```python
from build123d import *

# Parameters (mm, degrees)
MODEL_R                 = 1.5
SALIENTE_EXTRUIR1_DEPTH = 3


with BuildPart() as part:
    # Model → Saliente-Extruir1 (new body)
    with BuildSketch(Plane.XY):
        with BuildLine():
            Line((-1383.727545355, 378.908179756), (-1386.727545355, 378.908179756))
            Line((-1386.727545355, 378.908179756), (-1386.727545355, 380.408179756))
            ThreePointArc((-1386.727545355, 380.408179756), (-1387.166885184, 381.468839928), (-1388.227545355, 381.908179756))
            Line((-1388.227545355, 381.908179756), (-1395.72785056, 381.908179756))
            ThreePointArc((-1395.72785056, 381.908179756), (-1396.788510732, 381.468839928), (-1397.22785056, 380.408179756))
            Line((-1397.22785056, 380.408179756), (-1469.22785056, 380.408179756))
            ThreePointArc((-1469.22785056, 380.408179756), (-1469.667190388, 381.468839928), (-1470.72785056, 381.908179756))
            Line((-1470.72785056, 381.908179756), (-1478.227545355, 381.908179756))
            ThreePointArc((-1478.227545355, 381.908179756), (-1479.288205527, 381.468839928), (-1479.727545355, 380.408179756))
            Line((-1479.727545355, 380.408179756), (-1479.727545355, 378.908179756))
            Line((-1479.727545355, 378.908179756), (-1482.727545355, 378.908179756))
            Line((-1482.727545355, 378.908179756), (-1482.727545355, 368.408179756))
            Line((-1482.727545355, 368.408179756), (-1473.852545355, 368.408179756))
            Line((-1473.852545355, 368.408179756), (-1473.852545355, 369.658179757))
            ThreePointArc((-1473.852545355, 369.658179757), (-1473.632875441, 370.188509842), (-1473.102545355, 370.408179756))
            Line((-1473.102545355, 370.408179756), (-1471.352545355, 370.408179756))
            ThreePointArc((-1471.352545355, 370.408179756), (-1470.82221527, 370.188509842), (-1470.602545355, 369.658179757))
            Line((-1470.602545355, 369.658179757), (-1470.602545355, 368.408179756))
            Line((-1470.602545355, 368.408179756), (-1466.977545355, 368.408179756))
            ThreePointArc((-1466.977545355, 368.408179756), (-1466.44721527, 368.188509842), (-1466.227545355, 367.658179756))
            Line((-1466.227545355, 367.658179756), (-1466.227545355, 366.158179756))
            ThreePointArc((-1466.227545355, 366.158179756), (-1466.44721527, 365.627849671), (-1466.977545355, 365.408179756))
            Line((-1466.977545355, 365.408179756), (-1470.602545355, 365.408179756))
            Line((-1470.602545355, 365.408179756), (-1470.602545355, 364.158179756))
            ThreePointArc((-1470.602545355, 364.158179756), (-1470.82221527, 363.627849671), (-1471.352545355, 363.408179756))
            Line((-1471.352545355, 363.408179756), (-1473.102545355, 363.408179756))
            ThreePointArc((-1473.102545355, 363.408179756), (-1473.632875441, 363.627849671), (-1473.852545355, 364.158179756))
            Line((-1473.852545355, 364.158179756), (-1473.852545355, 365.408179756))
            Line((-1473.852545355, 365.408179756), (-1482.727545355, 365.408179756))
            Line((-1482.727545355, 365.408179756), (-1482.727545355, 350.408179756))
            Line((-1482.727545355, 350.408179756), (-1473.852545355, 350.408179756))
            Line((-1473.852545355, 350.408179756), (-1473.852545355, 351.658179756))
            ThreePointArc((-1473.852545355, 351.658179756), (-1473.632875441, 352.188509842), (-1473.102545355, 352.408179756))
            Line((-1473.102545355, 352.408179756), (-1471.352545355, 352.408179756))
            ThreePointArc((-1471.352545355, 352.408179756), (-1470.82221527, 352.188509842), (-1470.602545355, 351.658179756))
            Line((-1470.602545355, 351.658179756), (-1470.602545355, 350.408179756))
            Line((-1470.602545355, 350.408179756), (-1466.977545355, 350.408179756))
            ThreePointArc((-1466.977545355, 350.408179756), (-1466.44721527, 350.188509842), (-1466.227545355, 349.658179756))
            Line((-1466.227545355, 349.658179756), (-1466.227545355, 348.158179756))
            ThreePointArc((-1466.227545355, 348.158179756), (-1466.44721527, 347.627849671), (-1466.977545355, 347.408179756))
            Line((-1466.977545355, 347.408179756), (-1470.602545355, 347.408179756))
            Line((-1470.602545355, 347.408179756), (-1470.602545355, 346.158179756))
            ThreePointArc((-1470.602545355, 346.158179756), (-1470.82221527, 345.627849671), (-1471.352545355, 345.408179756))
            Line((-1471.352545355, 345.408179756), (-1473.102545355, 345.408179756))
            ThreePointArc((-1473.102545355, 345.408179756), (-1473.632875441, 345.627849671), (-1473.852545355, 346.158179756))
            Line((-1473.852545355, 346.158179756), (-1473.852545355, 347.408179756))
            Line((-1473.852545355, 347.408179756), (-1482.727545355, 347.408179756))
            Line((-1482.727545355, 347.408179756), (-1482.727545355, 336.908179756))
            Line((-1482.727545355, 336.908179756), (-1479.727545355, 336.908179756))
            Line((-1479.727545355, 336.908179756), (-1479.727545355, 335.408179756))
            ThreePointArc((-1479.727545355, 335.408179756), (-1479.288205527, 334.347519585), (-1478.227545355, 333.908179756))
            Line((-1478.227545355, 333.908179756), (-1470.72785056, 333.908179756))
            ThreePointArc((-1470.72785056, 333.908179756), (-1469.667190388, 334.347519585), (-1469.22785056, 335.408179756))
            Line((-1469.22785056, 335.408179756), (-1397.22785056, 335.408179756))
            ThreePointArc((-1397.22785056, 335.408179756), (-1396.788510732, 334.347519585), (-1395.72785056, 333.908179756))
            Line((-1395.72785056, 333.908179756), (-1388.227545355, 333.908179756))
            ThreePointArc((-1388.227545355, 333.908179756), (-1387.166885184, 334.347519585), (-1386.727545355, 335.408179756))
            Line((-1386.727545355, 335.408179756), (-1386.727545355, 336.908179756))
            Line((-1386.727545355, 336.908179756), (-1383.727545355, 336.908179756))
            Line((-1383.727545355, 336.908179756), (-1383.727545355, 347.408179756))
            Line((-1383.727545355, 347.408179756), (-1392.602545355, 347.408179756))
            Line((-1392.602545355, 347.408179756), (-1392.602545355, 346.158179756))
            ThreePointArc((-1392.602545355, 346.158179756), (-1392.82221527, 345.627849671), (-1393.352545355, 345.408179756))
            Line((-1393.352545355, 345.408179756), (-1395.102545355, 345.408179756))
            ThreePointArc((-1395.102545355, 345.408179756), (-1395.632875441, 345.627849671), (-1395.852545355, 346.158179756))
            Line((-1395.852545355, 346.158179756), (-1395.852545355, 347.408179756))
            Line((-1395.852545355, 347.408179756), (-1399.477545355, 347.408179756))
            ThreePointArc((-1399.477545355, 347.408179756), (-1400.007875441, 347.627849671), (-1400.227545355, 348.158179756))
            Line((-1400.227545355, 348.158179756), (-1400.227545355, 349.658179756))
            ThreePointArc((-1400.227545355, 349.658179756), (-1400.007875441, 350.188509842), (-1399.477545355, 350.408179756))
            Line((-1399.477545355, 350.408179756), (-1395.852545355, 350.408179756))
            Line((-1395.852545355, 350.408179756), (-1395.852545355, 351.658179756))
            ThreePointArc((-1395.852545355, 351.658179756), (-1395.632875441, 352.188509842), (-1395.102545355, 352.408179756))
            Line((-1395.102545355, 352.408179756), (-1393.352545355, 352.408179756))
            ThreePointArc((-1393.352545355, 352.408179756), (-1392.82221527, 352.188509842), (-1392.602545355, 351.658179756))
            Line((-1392.602545355, 351.658179756), (-1392.602545355, 350.408179756))
            Line((-1392.602545355, 350.408179756), (-1383.727545355, 350.408179756))
            Line((-1383.727545355, 350.408179756), (-1383.727545355, 365.408179756))
            Line((-1383.727545355, 365.408179756), (-1392.602545355, 365.408179756))
            Line((-1392.602545355, 365.408179756), (-1392.602545355, 364.158179756))
            ThreePointArc((-1392.602545355, 364.158179756), (-1392.82221527, 363.627849671), (-1393.352545355, 363.408179756))
            Line((-1393.352545355, 363.408179756), (-1395.102545355, 363.408179756))
            ThreePointArc((-1395.102545355, 363.408179756), (-1395.632875441, 363.627849671), (-1395.852545355, 364.158179756))
            Line((-1395.852545355, 364.158179756), (-1395.852545355, 365.408179756))
            Line((-1395.852545355, 365.408179756), (-1399.477545355, 365.408179756))
            ThreePointArc((-1399.477545355, 365.408179756), (-1400.007875441, 365.627849671), (-1400.227545355, 366.158179756))
            Line((-1400.227545355, 366.158179756), (-1400.227545355, 367.658179756))
            ThreePointArc((-1400.227545355, 367.658179756), (-1400.007875441, 368.188509842), (-1399.477545355, 368.408179756))
            Line((-1399.477545355, 368.408179756), (-1395.852545355, 368.408179756))
            Line((-1395.852545355, 368.408179756), (-1395.852545355, 369.658179757))
            ThreePointArc((-1395.852545355, 369.658179757), (-1395.632875441, 370.188509842), (-1395.102545355, 370.408179756))
            Line((-1395.102545355, 370.408179756), (-1393.352545355, 370.408179756))
            ThreePointArc((-1393.352545355, 370.408179756), (-1392.82221527, 370.188509842), (-1392.602545355, 369.658179757))
            Line((-1392.602545355, 369.658179757), (-1392.602545355, 368.408179756))
            Line((-1392.602545355, 368.408179756), (-1383.727545355, 368.408179756))
            Line((-1383.727545355, 368.408179756), (-1383.727545355, 378.908179756))
        make_face()
        with Locations((-1401.728155765, 357.908179756)):
            Circle(MODEL_R, mode=Mode.SUBTRACT)
        with Locations((-1464.728155765, 357.908179756)):
            Circle(MODEL_R, mode=Mode.SUBTRACT)
        with Locations((-1455.728155765, 357.908179756)):
            Circle(MODEL_R, mode=Mode.SUBTRACT)
        with Locations((-1410.728155765, 357.908179756)):
            Circle(MODEL_R, mode=Mode.SUBTRACT)
        with Locations((-1464.728155765, 375.908179756)):
            Circle(MODEL_R, mode=Mode.SUBTRACT)
        with Locations((-1455.728155765, 375.908179756)):
            Circle(MODEL_R, mode=Mode.SUBTRACT)
        with Locations((-1446.728155765, 375.908179756)):
            Circle(MODEL_R, mode=Mode.SUBTRACT)
        with Locations((-1437.728155765, 375.908179756)):
            Circle(MODEL_R, mode=Mode.SUBTRACT)
        with Locations((-1428.728155765, 375.908179756)):
            Circle(MODEL_R, mode=Mode.SUBTRACT)
        with Locations((-1419.728155765, 375.908179756)):
            Circle(MODEL_R, mode=Mode.SUBTRACT)
        with Locations((-1410.728155765, 375.908179756)):
            Circle(MODEL_R, mode=Mode.SUBTRACT)
        with Locations((-1401.728155765, 375.908179756)):
            Circle(MODEL_R, mode=Mode.SUBTRACT)
        with Locations((-1464.728155765, 339.908179757)):
            Circle(MODEL_R, mode=Mode.SUBTRACT)
        with Locations((-1455.728155765, 339.908179757)):
            Circle(MODEL_R, mode=Mode.SUBTRACT)
        with Locations((-1446.728155765, 339.908179757)):
            Circle(MODEL_R, mode=Mode.SUBTRACT)
        with Locations((-1437.728155765, 339.908179757)):
            Circle(MODEL_R, mode=Mode.SUBTRACT)
        with Locations((-1428.728155765, 339.908179757)):
            Circle(MODEL_R, mode=Mode.SUBTRACT)
        with Locations((-1419.728155765, 339.908179757)):
            Circle(MODEL_R, mode=Mode.SUBTRACT)
        with Locations((-1410.728155765, 339.908179757)):
            Circle(MODEL_R, mode=Mode.SUBTRACT)
        with Locations((-1401.728155765, 339.908179757)):
            Circle(MODEL_R, mode=Mode.SUBTRACT)
        with BuildLine():
            Line((-1448.227545355, 350.408179756), (-1418.227545355, 350.408179756))
            ThreePointArc((-1418.227545355, 350.408179756), (-1416.727545355, 348.908179756), (-1418.227545355, 347.408179756))
            Line((-1418.227545355, 347.408179756), (-1448.227545355, 347.408179756))
            ThreePointArc((-1448.227545355, 347.408179756), (-1449.727545355, 348.908179756), (-1448.227545355, 350.408179756))
        make_face(mode=Mode.SUBTRACT)
        with BuildLine():
            Line((-1448.227545355, 359.408179756), (-1418.227545355, 359.408179756))
            ThreePointArc((-1418.227545355, 359.408179756), (-1416.727545355, 357.908179756), (-1418.227545355, 356.408179756))
            Line((-1418.227545355, 356.408179756), (-1448.227545355, 356.408179756))
            ThreePointArc((-1448.227545355, 356.408179756), (-1449.727545355, 357.908179756), (-1448.227545355, 359.408179756))
        make_face(mode=Mode.SUBTRACT)
        with BuildLine():
            Line((-1448.227545355, 368.408179756), (-1418.227545355, 368.408179756))
            ThreePointArc((-1418.227545355, 368.408179756), (-1416.727545355, 366.908179756), (-1418.227545355, 365.408179756))
            Line((-1418.227545355, 365.408179756), (-1448.227545355, 365.408179756))
            ThreePointArc((-1448.227545355, 365.408179756), (-1449.727545355, 366.908179756), (-1448.227545355, 368.408179756))
        make_face(mode=Mode.SUBTRACT)
    extrude(amount=SALIENTE_EXTRUIR1_DEPTH)


solid = part.part
```
Check sheet for the modelled part. Datum: model origin and axes. Units: mm. A direction names the side the tool comes from. Round coordinates to 2 decimals unless told otherwise and drop trailing zeros. Order: outer loops, then holes, each group sorted by start corner. A loop starts at its lowest first (then second) coordinate and runs counter-clockwise, first axis right, second up. Notation, with made-up numbers: (36, 22.5) - (49, 22.5) arc R9 cw to (49, 37.5) - close; hole circle Ø9 at (48.5, -33). An arc over 180 degrees is marked (long way). Write item = value, one per line.
Q1. Draft check along X on faces 1 (the face through (-1482.728, 342, 1)), 2 (the face through (-1394, 370.408, 1)), 3 (the face through (-1437.036, 338.577, 1.479)), 4 (the face through (-1392, 333.908, 1)). Enter one of: pulls with the +X half, pulls with the -X half, needs draft (parallel to the pull), parting line crosses it, or undercut.
Computed:
face_1 = pulls with the -X half
face_2 = undercut
face_3 = undercut
face_4 = needs draft
Q2. Section check C-C (x = -1419.5). Record the boundary of the cut face in (y, z), and give its area (3 significant figures).
Computed:
outline = (335.41, 0) - (338.43, 0) - (338.43, 3) - (335.41, 3) - close; (341.39, 0) - (347.41, 0) - (347.41, 3) - (341.39, 3) - close; (350.41, 0) - (356.41, 0) - (356.41, 3) - (350.41, 3) - close; (359.41, 0) - (365.41, 0) - (365.41, 3) - (359.41, 3) - close; (368.41, 0) - (374.43, 0) - (374.43, 3) - (368.41, 3) - close; (377.39, 0) - (380.41, 0) - (380.41, 3) - (377.39, 3) - close
area = 90.2 mm^2
Q3. Section check B-B (x = -1434.5). Record the boundary of the cut face in (y, z).
Computed:
outline = (335.41, 0) - (347.41, 0) - (347.41, 3) - (335.41, 3) - close; (350.41, 0) - (356.41, 0) - (356.41, 3) - (350.41, 3) - close; (359.41, 0) - (365.41, 0) - (365.41, 3) - (359.41, 3) - close; (368.41, 0) - (380.41, 0) - (380.41, 3) - (368.41, 3) - close
Q4. Thickness scan on line 1 along Y through (x, z) = (-1434, 0.4); line 2 along Y through (x, z) = (-1401.5, 2.75); line 3 along Y through (x, z) = (-1437, 1.85). Record the ranges inside material, lowest first.
Computed:
line_1 = 335.41 to 347.41, 350.41 to 356.41, 359.41 to 365.41, 368.41 to 380.41
line_2 = 335.41 to 338.43, 341.39 to 356.43, 359.39 to 374.43, 377.39 to 380.41
line_3 = 335.41 to 338.6, 341.22 to 347.41, 350.41 to 356.41, 359.41 to 365.41, 368.41 to 374.6, 377.22 to 380.41
Q5. Tool access check on faces 5 (the face through (-1449.727, 348.875, 1.479)), 6 (the face through (-1469, 365.408, 1)), 7 (the face through (-1398, 365.408, 1)), 8 (the face through (-1482.728, 358, 1)). Record the directions out of +Z, -Z, +X, -X, +Y, -Y that give a thin tool (end or side, any length) a straight path to the whole face; none if there is none.
Computed:
face_5 = +Z, -Z
face_6 = +Z, -Z, -X
face_7 = +Z, -Z, +X
face_8 = +Z, -Z, -X, +Y, -Y
Q6. Go/stop test with flat-tipped pins: pin 1 (1 mm diameter, centred on x = -1439.5, z = 0.5, fed in from -Y); pin 2 (1.2 mm diameter, centred on y = 367, z = 2, fed in from +X); pin 3 (2.5 mm diameter, centred on x = -1437.73, y = 375.91, fed in from +Z). Record where each tip stops, or that it passes through.
Computed:
pin_1 = 335.41
pin_2 = -1400.23
pin_3 = through
Q7. Section check D-D (x = -1405.5). Record the boundary of the cut face in (y, z), and give its area (3 significant figures).
Computed:
outline = (335.41, 0) - (380.41, 0) - (380.41, 3) - (335.41, 3) - close
area = 135 mm^2
Q8. Section check A-A (x = -1390.5). Record the boundary of the cut face in (y, z), and give its area (3 significant figures).
Computed:
outline = (333.91, 0) - (347.41, 0) - (347.41, 3) - (333.91, 3) - close; (350.41, 0) - (365.41, 0) - (365.41, 3) - (350.41, 3) - close; (368.41, 0) - (381.91, 0) - (381.91, 3) - (368.41, 3) - close
area = 126 mm^2
